Can you work these out from the model? Positions are in its coordinate system, mm. Face numbers are marked on the shaded views. A direction names the side the tool comes from. Give positions to 0.01 mm unless a question says otherwise; leave off trailing zeros. Write each loop counter-clockwise with the first axis right and the second up, starting at its lowest first coordinate (ties: lowest second). Pieces come first, ordered by that corner, then holes.
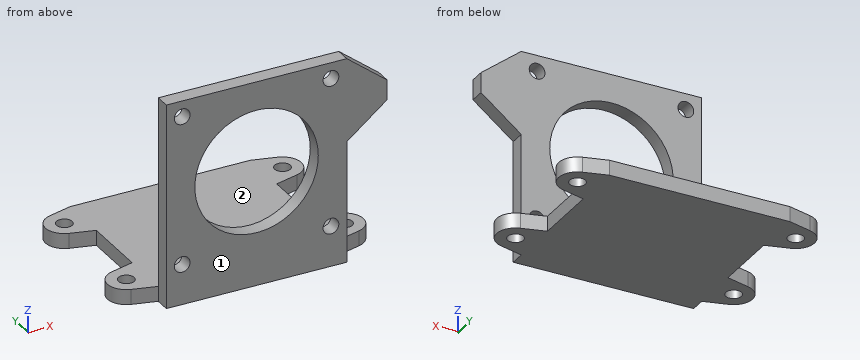
from build123d import *

# Parameters (mm, degrees)
SKETCH1_W              = 57
SKETCH1_H              = 57
BOSS_EXTRUDE1_DEPTH    = 4.7625
SKETCH2_W              = 57
SKETCH2_H              = 4.7625
BOSS_EXTRUDE2_DEPTH    = 60
SKETCH3_R              = 19.5
CUT_EXTRUDE1_DEPTH     = 5.7625
F_10_CLEARANCE_HOLE1_D = 4.9784
BOSS_EXTRUDE3_DEPTH    = 4.7625
F_10_CLEARANCE_HOLE2_D = 4.9784
BOSS_EXTRUDE4_DEPTH    = 4.7625


with BuildPart() as part:
    # Sketch1 → Boss-Extrude1 (new body)
    with BuildSketch(Plane.XY):
        Rectangle(SKETCH1_W, SKETCH1_H)
    extrude(amount=BOSS_EXTRUDE1_DEPTH)

    # Sketch2 → Boss-Extrude2 (add)
    with BuildSketch(Plane.XY.offset(4.7625)):
        with Locations((0, -26.11875)):
            Rectangle(SKETCH2_W, SKETCH2_H)
    extrude(amount=BOSS_EXTRUDE2_DEPTH)

    # Sketch3 → Cut-Extrude1 (cut, through all)
    with BuildSketch(Plane(origin=(0, -23.7375, 0), x_dir=(1, 0, 0), z_dir=(0, 1, 0))):
        with Locations((0, -36.2625)):
            Circle(SKETCH3_R)
    extrude(amount=-CUT_EXTRUDE1_DEPTH, mode=Mode.SUBTRACT)

    # #10 Clearance Hole1 (through all)
    with Locations(Plane(origin=(0, -28.5, 0), x_dir=(-1, 0, 0), z_dir=(0, -1, 0))):
        with Locations((0, -36.2625), (-23.495, -12.7675), (23.495, -59.7575), (23.495, -12.7675), (-23.495, -59.7575)):
            Hole(F_10_CLEARANCE_HOLE1_D / 2)

    # Sketch7 → Boss-Extrude3 (add)
    with BuildSketch(Plane.XY):
        with BuildLine():
            Line((28.5, -23.7375), (35.993907128, -21.729513637))
            ThreePointArc((35.993907128, -21.729513637), (40.40625, -15.979236452), (35.993907128, -10.228959268))
            Line((35.993907128, -10.228959268), (28.5, -8.220972905))
            Line((28.5, -8.220972905), (28.5, -23.7375))
        make_face()
        with BuildLine():
            Line((28.5, 12.983472905), (35.993907128, 14.991459268))
            ThreePointArc((35.993907128, 14.991459268), (40.40625, 20.741736452), (35.993907128, 26.492013637))
            Line((35.993907128, 26.492013637), (28.5, 28.5))
            Line((28.5, 28.5), (28.5, 12.983472905))
        make_face()
        with BuildLine():
            Line((-28.5, 28.5), (-28.5, 12.983472905))
            Line((-28.5, 12.983472905), (-35.993907128, 14.991459268))
            ThreePointArc((-35.993907128, 14.991459268), (-40.40625, 20.741736452), (-35.993907128, 26.492013637))
            Line((-35.993907128, 26.492013637), (-28.5, 28.5))
        make_face()
        with BuildLine():
            Line((-28.5, -23.7375), (-35.993907128, -21.729513637))
            ThreePointArc((-35.993907128, -21.729513637), (-40.40625, -15.979236452), (-35.993907128, -10.228959268))
            Line((-35.993907128, -10.228959268), (-28.5, -8.220972905))
            Line((-28.5, -8.220972905), (-28.5, -23.7375))
        make_face()
    extrude(amount=BOSS_EXTRUDE3_DEPTH)

    # #10 Clearance Hole2 (through all)
    with Locations(Plane.XY.offset(4.7625)):
        with Locations((34.453125, -15.979236452), (34.453125, 20.741736452), (-34.453125, 20.741736452), (-34.453125, -15.979236452)):
            Hole(F_10_CLEARANCE_HOLE2_D / 2)

    # Sketch10 → Boss-Extrude4 (add)
    with BuildSketch(Plane.XZ.offset(28.5)):
        Polygon((41.2, 48.3795), (41.2, 54.7295), (28.5, 64.7625), (28.5, 38.3465), align=None)
    extrude(amount=-BOSS_EXTRUDE4_DEPTH)


solid = part.part
(1) Will these pins go through, and if not, where does the flat tip stop? P1, Ø2.5, axis at y = 7.5, z = 3.5, coming from the -X side; P2, Ø8, axis at x = -34.45, y = -15.98, coming from the +Z side; P3, Ø2.5, axis at y = -26.5, z = 12.5, coming from the +X side; P4, Ø3, axis at x = 34.45, y = -15.98, coming from the -Z side.
Returned:
P1: stops at x = -28.5
P2: stops at z = 4.76
P3: stops at x = 28.5
P4: passes through
(2) Imagine slicing it at B-B, the plane x = 5. Write out the boundary of the cut face in (y, z).
Returned:
outline: (-28.5, 0) - (28.5, 0) - (28.5, 4.76) - (-23.74, 4.76) - (-23.74, 17.41) - (-28.5, 17.41) - close; (-28.5, 55.11) - (-23.74, 55.11) - (-23.74, 64.76) - (-28.5, 64.76) - close
(3) Imagine slicing it at D-D, the plane x = -30.5. Write out the boundary of the cut face in (y, z).
Returned:
outline: (-23.2, 0) - (-8.76, 0) - (-8.76, 4.76) - (-23.2, 4.76) - close; (13.52, 0) - (27.96, 0) - (27.96, 4.76) - (13.52, 4.76) - close
(4) For the marked faces 1 and 2, which set-ups out of +Z, -Z, +X, -X, +Y, -Y let a thin tool reach every point of the face, with its end or its side?
Returned:
face 1: +Z, -Z, +X, -X, -Y
face 2: +Z, +X, -X, +Y
(5) Imagine slicing it at A-A, the plane z = 24.5. Write out the boundary of the cut face in (x, y), plus the area to 3 significant figures.
Returned:
outline: (-28.5, -28.5) - (-15.55, -28.5) - (-15.55, -23.74) - (-28.5, -23.74) - close; (15.55, -28.5) - (28.5, -28.5) - (28.5, -23.74) - (15.55, -23.74) - close
area: 123 mm2
(6) If I drill on L1, parallel to Z at x = 25, y = 18.5; L2, parallel to Y at x = -17, z = 16; L3, parallel to Z at x = 0, y = -24.85, over which ranges is the centre line in solid material (lowest first)?
Returned:
L1: z = 0 to 4.76
L2: y = -28.5 to -23.74
L3: z = 0 to 16.76, 55.76 to 64.76
(7) Imagine slicing it at C-C, the plane y = 12. Write out the boundary of the cut face in (x, z).
Returned:
outline: (-28.5, 0) - (28.5, 0) - (28.5, 4.76) - (-28.5, 4.76) - close
